```python
from build123d import *

# Parameters (mm, degrees)
F0_W     = 19.05
F0_H     = 19.05
F0_W_2   = 15.8623
F0_H_2   = 15.8623
F1_DEPTH = 438.15
F2_R     = 3.1242
F3_DEPTH = 19.051


with BuildPart() as f1:
    # F0 (on Front) → F1 (new body)
    with BuildSketch(Plane.XZ):
        with Locations((-0.55224, -2.118741)):
            Rectangle(F0_W, F0_H)
        with Locations((-0.54589, -2.112391)):
            Rectangle(F0_W_2, F0_H_2, mode=Mode.SUBTRACT)
    extrude(amount=F1_DEPTH)

    # F2 (on face) → F3 (cut, through all)
    with BuildSketch(Plane.XY.offset(7.406259)):
        with Locations((-0.55224, -10.16508)):
            Circle(F2_R)
        with Locations((-0.55224, -428.80788)):
            Circle(F2_R)
    extrude(amount=-F3_DEPTH, mode=Mode.SUBTRACT)


solid = f1.part
```
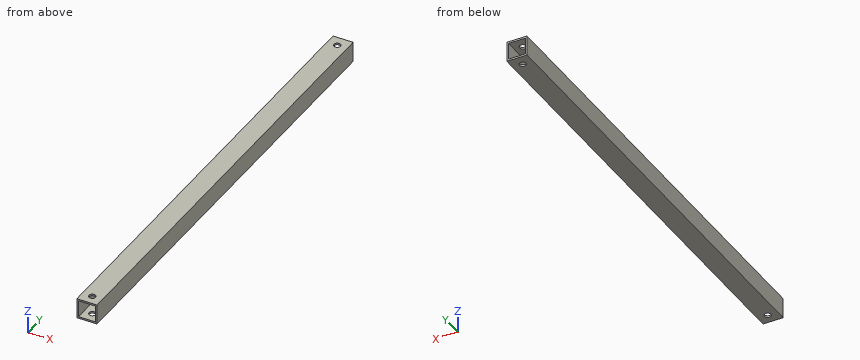
Check sheet for the modelled part. Datum: model origin and axes. Units: mm. Coordinates: 2 decimals unless noted, no trailing zeros. Write each loop counter-clockwise with the first axis right and the second up, starting at its lowest first coordinate (ties: lowest second). Pieces come first, ordered by that corner, then holes. Notation, with made-up numbers: (80.5, 64) -> (130.5, 64) arc R3 ccw to (130.5, 69) -> close; hole circle Ø10 at (68, -29). An arc over 180 degrees is marked (long way). Use a Markdown table: item, result.
1. Sectioned sample at A-A (z = -1.75). Enter the section's corners in (x, y), plus the area to 3 significant figures.
Reported:
| item | result |
|---|---|
| outline | (-10.08, -438.15) -> (-8.48, -438.15) -> (-8.48, 0) -> (-10.08, 0) -> close; (7.39, -438.15) -> (8.97, -438.15) -> (8.97, 0) -> (7.39, 0) -> close |
| area | 1,400 mm2 |
2. Sectioned sample at B-B (y = -154.5). Enter the section's corners in (x, z).
Reported:
| item | result |
|---|---|
| outline | (-10.08, -11.64) -> (8.97, -11.64) -> (8.97, 7.41) -> (-10.08, 7.41) -> close; hole (-8.48, -10.04) -> (7.39, -10.04) -> (7.39, 5.82) -> (-8.48, 5.82) -> close |
3. Scan lines: line 1 along Z through (x, y) = (-6.5, -375); line 2 along X through (y, z) = (-259, -4.75). Record each from-to range of solid material in increasing order.
Reported:
| item | result |
|---|---|
| line 1 | z = -11.64 to -10.04, 5.82 to 7.41 |
| line 2 | x = -10.08 to -8.48, 7.39 to 8.97 |
